Input: part model. Units: mm. Frame: model coordinates. Round coordinates to 2 decimals unless told otherwise and drop trailing zeros. Loops run counter-clockwise (first coordinate to the right, second up) from the corner with the lowest first, then second, coordinate; pieces in that order, holes last. Notation, with made-up numbers: (84, 2.25) -> (126, 2.25) arc R15 ccw to (126, 26.25) -> close; hole circle Ø7 at (61.25, -9). An arc over 180 degrees is marked (long way). Answer as a JSON object with one key per item and string values. Group by question number.
Item 1: Pin query (flat end, axial travel): pin 1 (1.8 mm diameter, centred on x = -45.51, y = 24.09, fed in from -Z). Return the tip coordinate at first contact, or that it passes through.
Item 2: Section query B-B on z = 1.6. Count the separate pieces of the cut face and the enclosed holes in it, and give its area (3 significant figures).
Item 3: Material intervals for line 1 (X direction, y = 27, z = 1.5); line 2 (X direction, y = 29, z = 0.4); line 3 (Y direction, x = -71, z = 1.2), sorted ascending. Write a range as [from, to].
Item 4: Draft query along Y for faces 1 (the cylindrical face through (23.639, 23.464, 1.014)), 2 (the flat face through (-5, 28, 0)), 3 (the cylindrical face through (56.053, 25.448, 1.014)). Return one class per face: released by +Y, released by -Y, zero draft, split by the parting line, or undercut.
Item 5: Section query A-A on x = 66. Return loops of the section in (y, z).
from build123d import *

# Parameters (mm, degrees)
SKETCH_5_W          = 206
SKETCH_5_H          = 45
EXTRUDE_3_DEPTH     = 2
SKETCH_6_R          = 11
SKETCH_6_R_2        = 1.474928536
SKETCH_6_R_3        = 1.25
SKETCH_6_R_4        = 4.75
SKETCH_6_R_5        = 5.5
SKETCH_6_W          = 9.6
SKETCH_6_H          = 8.3
SKETCH_6_W_2        = 12
SKETCH_6_H_2        = 11
CUT_EXTRUDE_1_DEPTH = 10
SKETCH_1_R          = 1.25
CUT_EXTRUDE_7_DEPTH = 70
FILLET_1_R          = 1


with BuildPart() as part:
    # Sketch 5 → Extrude 3 (new body)
    with BuildSketch(Plane.XY):
        with Locations((-3.884539257, 17.589033065)):
            Rectangle(SKETCH_5_W, SKETCH_5_H)
    extrude(amount=EXTRUDE_3_DEPTH)

    # Sketch 6 → Cut-Extrude 1 (cut)
    with BuildSketch(Plane.XY.offset(2)):
        with Locations((-62.284539257, 14.189033065)):
            Circle(SKETCH_6_R)
        with Locations((-35.614539257, 14.189033065)):
            Circle(SKETCH_6_R)
        with Locations((-8.944539257, 14.189033065)):
            Circle(SKETCH_6_R)
        with Locations((17.725460743, 14.189033065)):
            Circle(SKETCH_6_R)
        with Locations((-72.184539257, 24.089033065)):
            Circle(SKETCH_6_R_2)
        with Locations((-52.384539257, 4.289033065)):
            Circle(SKETCH_6_R_2)
        with Locations((-45.514539257, 24.089033065)):
            Circle(SKETCH_6_R_2)
        with Locations((-25.714539257, 4.289033065)):
            Circle(SKETCH_6_R_2)
        with Locations((-18.844539257, 24.089033065)):
            Circle(SKETCH_6_R_2)
        with Locations((0.955460743, 4.289033065)):
            Circle(SKETCH_6_R_2)
        with Locations((7.825460743, 24.089033065)):
            Circle(SKETCH_6_R_2)
        with Locations((27.625460743, 4.289033065)):
            Circle(SKETCH_6_R_2)
        with Locations((37.665460743, 17.739033065)):
            Circle(SKETCH_6_R_3)
        with Locations((51.185460743, 17.739033065)):
            Circle(SKETCH_6_R_3)
        with Locations((51.665460743, 27.26693986)):
            Circle(SKETCH_6_R_4)
        with Locations((37.665460743, 27.26693986)):
            Circle(SKETCH_6_R_4)
        with Locations((-86.884539257, 27.26693986)):
            Circle(SKETCH_6_R_5)
        with Locations((-86.884539257, 10.74540099)):
            Circle(SKETCH_6_R_5)
        with Locations((37.665460743, 7.739033065)):
            Rectangle(SKETCH_6_W, SKETCH_6_H)
        with Locations((51.185460743, 7.739033065)):
            Rectangle(SKETCH_6_W, SKETCH_6_H)
        with Locations((66.825460743, 7.189033065)):
            Rectangle(SKETCH_6_W_2, SKETCH_6_H_2)
    extrude(amount=-CUT_EXTRUDE_1_DEPTH, mode=Mode.SUBTRACT)

    # Sketch 1 → Cut-Extrude 7 (cut)
    with BuildSketch(Plane.XY):
        with Locations((-100.384539257, 35.089033065)):
            Circle(SKETCH_1_R)
        with Locations((-100.384539257, 0.089033065)):
            Circle(SKETCH_1_R)
        with Locations((92.615460743, 0.089033065)):
            Circle(SKETCH_1_R)
        with Locations((92.615460743, 35.089033065)):
            Circle(SKETCH_1_R)
    extrude(amount=CUT_EXTRUDE_7_DEPTH, mode=Mode.SUBTRACT)

    # Fillet 1
    fillet_1_edges = [part.edges().sort_by_distance(p)[0] for p in [
        (-106.884539257, -4.910966935, 1),
        (-106.884539257, 40.089033065, 1),
        (99.115460743, 40.089033065, 1),
        (99.115460743, -4.910966935, 1),
    ]]
    fillet(fillet_1_edges, radius=FILLET_1_R)


solid = part.part
Solved:
{
 "1": {"pin 1": "through"},
 "2": {"separate pieces": "1", "enclosed holes": "25", "area": "7,040 mm²"},
 "3": {"line 1": "[-106.88, -92.38], [-81.39, 32.92], [42.41, 46.92], [56.41, 99.12]", "line 2": "[-106.88, -92.1], [-81.66, 33.24], [42.09, 47.24], [56.09, 99.12]", "line 3": "[-4.91, 7.48], [20.9, 23.21], [24.97, 40.09]"},
 "4": {"face 1": "undercut", "face 2": "zero draft", "face 3": "undercut"},
 "5": {"outline": "(-4.91, 0) -> (1.69, 0) -> (1.69, 2) -> (-4.91, 2) -> close; (12.69, 0) -> (40.09, 0) -> (40.09, 2) -> (12.69, 2) -> close"}
}
